Design review of the part built by this model. Coordinates are the model's own, in mm. A direction names the side the tool comes from. Coordinates: 2 decimals unless noted, no trailing zeros. Order: outer loops, then holes, each group sorted by start corner. A loop starts at its lowest first (then second) coordinate and runs counter-clockwise, first axis right, second up. Notation, with made-up numbers: M 67,-1 L 125,-1 A11 ccw 125,7 Z; hole C -38.5,48.25 d7. An arc over 180 degrees is marked long. Answer as a JSON object with one key per item and string values.
from build123d import *

# Parameters (mm, degrees)
F0_R     = 4
F1_DEPTH = 5
F2_W     = 10
F2_H     = 2
F3_DEPTH = 24.001
F4_R     = 1


with BuildPart() as f1:
    # F0 (on Front) → F1 (new body)
    with BuildSketch(Plane.XZ):
        with BuildLine():
            Line((14.836441, 12), (-21.763559, 12))
            ThreePointArc((-21.763559, 12), (-33.763559, 0), (-21.763559, -12))
            Line((-21.763559, -12), (14.836441, -12))
            ThreePointArc((14.836441, -12), (26.836441, 0), (14.836441, 12))
        make_face()
        with Locations((-21.763559, 0)):
            Circle(F0_R, mode=Mode.SUBTRACT)
        with Locations((14.836441, 0)):
            Circle(F0_R, mode=Mode.SUBTRACT)
    extrude(amount=F1_DEPTH)

    # F2 (on face) → F3 (cut, through all)
    with BuildSketch(Plane.XY.offset(12)):
        with Locations((2.836441, -1)):
            Rectangle(F2_W, F2_H)
    extrude(amount=-F3_DEPTH, mode=Mode.SUBTRACT)

    # F4
    f4_edges = [f1.edges().sort_by_distance(p)[0] for p in [
        (7.836441, -2, 0),
        (-2.163559, -2, 0),
    ]]
    fillet(f4_edges, radius=F4_R)


solid = f1.part
1) Mouldability with a two-part tool opening along X and no side actions: class faces 1 (the cylindrical face through (16.68, -2.46, -3.55)), 2 (the flat face through (-4, -5, 0)), 3 (the cylindrical face through (26.834, -2.465, -0.264)) as released by +X, released by -X, zero draft, split by the parting line, or undercut.
Taken from the geometry:
{"face 1": "undercut", "face 2": "zero draft", "face 3": "released by +X"}
2) To check wall thickness, follow L1, parallel to X at y = -1.5, z = 1; L2, parallel to Y at x = 7, z = 4.5; L3, parallel to X at y = -1.7, z = -10.75. State the ranges of each line that lie inside material, in increasing order.
Taken from the geometry:
{"L1": "x = -33.72 to -25.64, -17.89 to -2.03, 7.7 to 10.96, 18.71 to 26.79", "L2": "y = -5 to -1.99", "L3": "x = -27.1 to -1.88, 7.55 to 20.17"}
3) Tool access review of faces 4 (the flat face through (-2.164, -0.5, 0.2)), 5 (the cylindrical face through (-25.76, -2.46, 0.18)): name each direction out of +Z, -Z, +X, -X, +Y, -Y from which nothing blocks a thin tool from reaching the whole face with its end or side.
Taken from the geometry:
{"face 4": "+Z, -Z, +Y", "face 5": "+Y, -Y"}
4) Insertion check: pin 1 Ø0.5 at (y, z) = (-0.5, 5) entering from +X; pin 2 Ø0.5 at (y, z) = (-0.5, -4) entering from -X; pin 3 Ø4 at (x, z) = (1, -3.5) entering from +Y; pin 4 Ø7 at (x, z) = (14.84, 0) entering from +Y. Each pin has a flat end and moves straight along its axis. Give the tip position at first contact, or say it passes through.
Taken from the geometry:
{"pin 1": "stops at x = 25.86", "pin 2": "stops at x = -33.16", "pin 3": "stops at y = -2", "pin 4": "passes through"}
5) Add section B-B (x = 0). State the section outline as (y, z) points, and give its area (3 significant figures).
Taken from the geometry:
{"outline": "M -5,-12 L -2,-12 L -2,12 L -5,12 Z", "area": "72.0 mm2"}
6) Add section A-A (z = 0). State the section outline as (x, y) points.
Taken from the geometry:
{"outline": "M -33.76,-5 L -25.76,-5 L -25.76,0 L -33.76,0 Z; M -17.76,-5 L 10.84,-5 L 10.84,0 L 7.84,0 L 7.84,-1 A1 cw 6.84,-2 L -1.16,-2 A1 cw -2.16,-1 L -2.16,0 L -17.76,0 Z; M 18.84,-5 L 26.84,-5 L 26.84,0 L 18.84,0 Z"}
7) Add section C-C (x = -29.5). State the section outline as (y, z) points, and give its area (3 significant figures).
Taken from the geometry:
{"outline": "M -5,-9.17 L 0,-9.17 L 0,9.17 L -5,9.17 Z", "area": "91.7 mm2"}
